Drawing for the job (mm, zero at the part's lowest x, y, z). A direction names the side the tool comes from. Round coordinates to 2 decimals unless told otherwise and drop trailing zeros. Write each loop counter-clockwise with the first axis right and the second up, starting at its lowest first coordinate (ties: lowest second). Pieces come first, ordered by that corner, then holes.
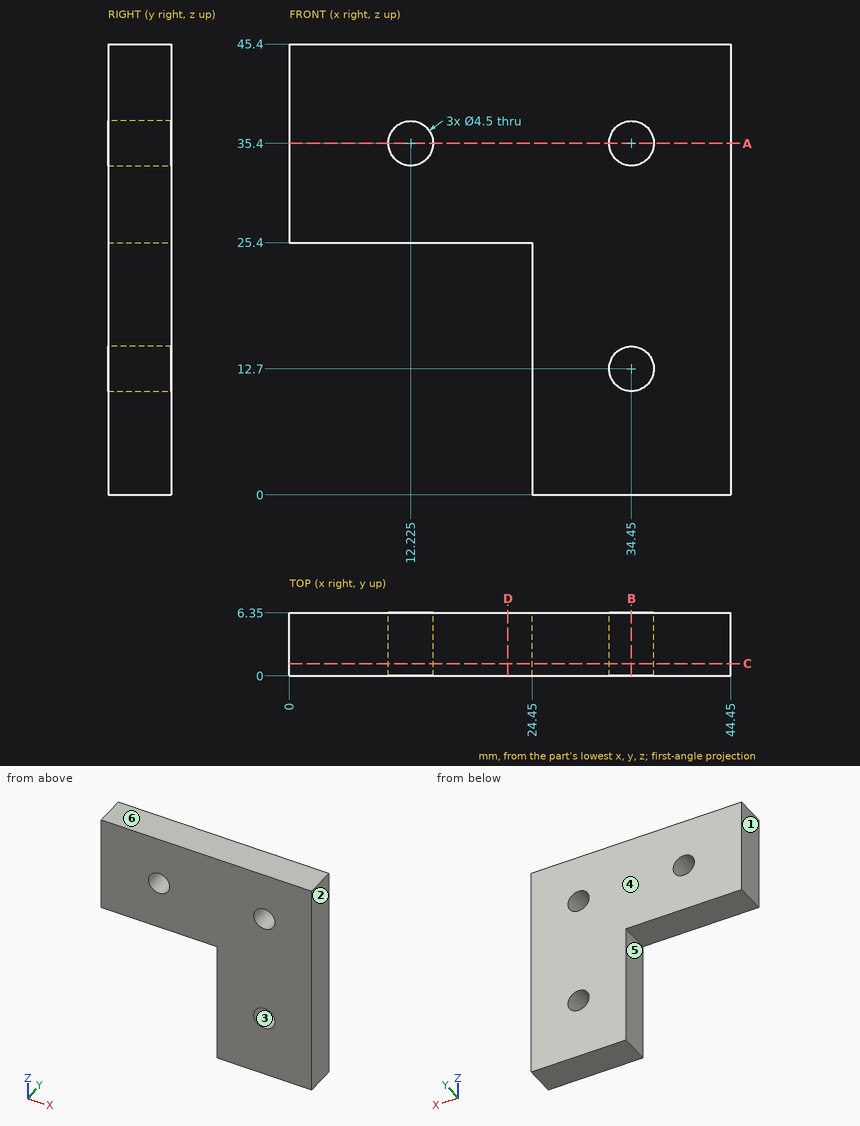
1) Which spindle directions (+Z, -Z, +X, -X, +Y, -Y) get a long thin tool onto all of the face, cutting with end or side? Do the marked faces 5 and 6. Say none if no direction does.
2) Cut at D-D on x = 22. List the corners of the cut face in (y, z), and give its area (3 significant figures).
3) Pull direction X, two halves, no side cores. Call the marked faces 1, 2, 3 and 4: released by +X, released by -X, zero draft, split by the parting line, or undercut.
4) Cut at B-B on x = 34.45. List the corners of the cut face in (y, z), and give its area (3 significant figures).
5) Flat gauge pins, fed straight in: pin 1 Ø3.5 at (x, z) = (34.45, 35.4) entering from -Y; pin 2 Ø3 at (y, z) = (2.5, 16) entering from -X. Where does each tip first touch, or does it go through?
6) Cut at C-C on y = 1.25. List the corners of the cut face in (x, z) (3 decimals), and give its area (3 significant figures).
7) Cut at A-A on z = 35.4. List the corners of the cut face in (x, y) (3 decimals), and give its area (3 significant figures).
8) Wall check: probe 1 along X at (y, z) = (1.75, 35.4) (3 decimals); probe 2 along Z at (x, y) = (35.5, 2.5); probe 3 along X at (y, z) = (5.5, 35). Give the ranges that are in metal, low to high.
Result sheet:
1. face 5: -Z, -X, +Y, -Y
1. face 6: +Z, +X, -X, +Y, -Y
2. outline: (0, 25.4) - (6.35, 25.4) - (6.35, 45.4) - (0, 45.4) - close
2. area: 127 mm2
3. face 1: released by -X
3. face 2: released by +X
3. face 3: undercut
3. face 4: zero draft
4. outline: (0, 0) - (6.35, 0) - (6.35, 10.45) - (0, 10.45) - close; (0, 14.95) - (6.35, 14.95) - (6.35, 33.15) - (0, 33.15) - close; (0, 37.65) - (6.35, 37.65) - (6.35, 45.4) - (0, 45.4) - close
4. area: 231 mm2
5. pin 1: passes through
5. pin 2: stops at x = 24.45
6. outline: (0, 25.4) - (24.45, 25.4) - (24.45, 0) - (44.45, 0) - (44.45, 45.4) - (0, 45.4) - close; hole circle Ø4.5 at (12.225, 35.4); hole circle Ø4.5 at (34.45, 12.7); hole circle Ø4.5 at (34.45, 35.4)
6. area: 1,350 mm2
7. outline: (0, 0) - (9.975, 0) - (9.975, 6.35) - (0, 6.35) - close; (14.475, 0) - (32.2, 0) - (32.2, 6.35) - (14.475, 6.35) - close; (36.7, 0) - (44.45, 0) - (44.45, 6.35) - (36.7, 6.35) - close
7. area: 225 mm2
8. probe 1: x = 0 to 9.975, 14.475 to 32.2, 36.7 to 44.45
8. probe 2: z = 0 to 10.71, 14.69 to 33.41, 37.39 to 45.4
8. probe 3: x = 0 to 10.01, 14.44 to 32.24, 36.66 to 44.45
